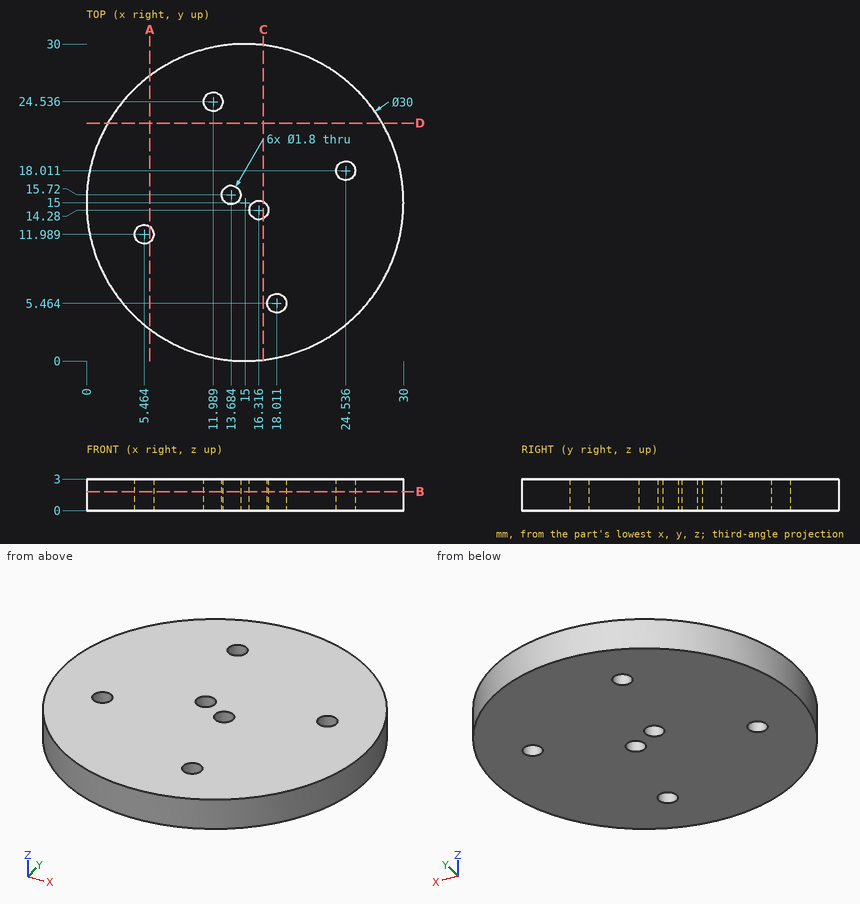
Design review of the part shown in the three views and the two pictorial views. Dimensions are in mm from the part's minimum x, y and z. Give positions to 0.01 mm unless a question says otherwise; leave off trailing zeros. Order: outer loops, then holes, each group sorted by start corner. A loop starts at its lowest first (then second) coordinate and runs counter-clockwise, first axis right, second up. Notation, with made-up numbers: M 21.25,76.25 L 25.25,76.25 A18 cw 25.25,107.25 Z; hole C 50,80.5 d5. An arc over 180 degrees is marked long. Answer in a Markdown table with one row per item. Add a question column.
(1) Consider section A-A on x = 6. State the section outline as (y, z) points.
(2) Consider section C-C on x = 16.75. State the section outline as (y, z) points.
(3) Wall thickness on probe 1 along Y at (x, z) = (24.75, 1.8) (1 decimal); probe 2 along Y at (x, z) = (17, 0.55) (1 decimal); probe 3 along X at (y, z) = (13.75, 1.15): over which ranges is each line inside the solid? List them lowest first. Write a range as [from, to].
(4) Consider section B-B on z = 1.8. State the section outline as (x, y) points.
(5) Consider section D-D on y = 22.5. State the section outline as (x, z) points.
Evaluation:
| question | item | result |
|---|---|---|
| 1 | outline | M 3,0 L 11.27,0 L 11.27,3 L 3,3 Z; M 12.71,0 L 27,0 L 27,3 L 12.71,3 Z |
| 2 | outline | M 0.1,0 L 13.49,0 L 13.49,3 L 0.1,3 Z; M 15.07,0 L 29.9,0 L 29.9,3 L 15.07,3 Z |
| 3 | probe 1 | y = [3.6, 17.1], [18.9, 26.4] |
| 3 | probe 2 | y = [0.1, 13.7], [14.9, 29.9] |
| 3 | probe 3 | x = [0.05, 15.59], [17.04, 29.95] |
| 4 | outline | C 15,15 d30; hole C 5.46,11.99 d1.8; hole C 11.99,24.54 d1.8; hole C 13.68,15.72 d1.8; hole C 16.32,14.28 d1.8; hole C 18.01,5.46 d1.8; hole C 24.54,18.01 d1.8 |
| 5 | outline | M 2.01,0 L 27.99,0 L 27.99,3 L 2.01,3 Z |
